For this review, use the dimensioned drawing (mm, ordinates from the lowest corner) and the shaded views. A direction names the side the tool comes from. Give positions to 0.01 mm unless a question says otherwise; leave off trailing zeros. Write each loop counter-clockwise with the first axis right and the second up, starting at its lowest first coordinate (ties: lowest second). Pieces come first, ordered by that corner, then holes.
1) We need section A-A on z = 2. Give the boundary of the cut face in (x, y).
2) We need section D-D on y = 16.5. Give the boundary of the cut face in (x, z), and give its area (3 significant figures).
3) We need section C-C on x = 10.25. Give the boundary of the cut face in (y, z).
4) We need section B-B on x = 5. Give the number of separate pieces and of enclosed holes in the cut face, and give its area (3 significant figures).
5) Machinability: for the marked faces 5, 6, 7, 8 and 9, which of the approach directions +Z, -Z, +X, -X, +Y, -Y give a long, thin tool a straight path to every point of the face, cutting with its end or side? Answer none if there is none.
6) For P1, Ø2, axis at x = 8.5, z = 9, coming from the -Y side; P2, Ø4, axis at x = 8, y = 27.5, coming from the -Z side; P3, Ø0.8, axis at x = 2, z = 13, coming from the -Y side, all flat-tipped, find the tip position at first contact; note any pin that passes through.
7) Wall thickness on line 1 along Z through (x, y) = (5, 31); line 2 along Z through (x, y) = (2.25, 19); line 3 along X through (y, z) = (15, 9.5): over which ranges is each line inside the solid? List them lowest first.
8) Draft analysis for pull direction Y (two halves, no side actions). For the marked faces 1, 2, 3 and 4, state which applies: pulls with the +Y half, pulls with the -Y half, needs draft (parallel to the pull), parting line crosses it, or undercut.
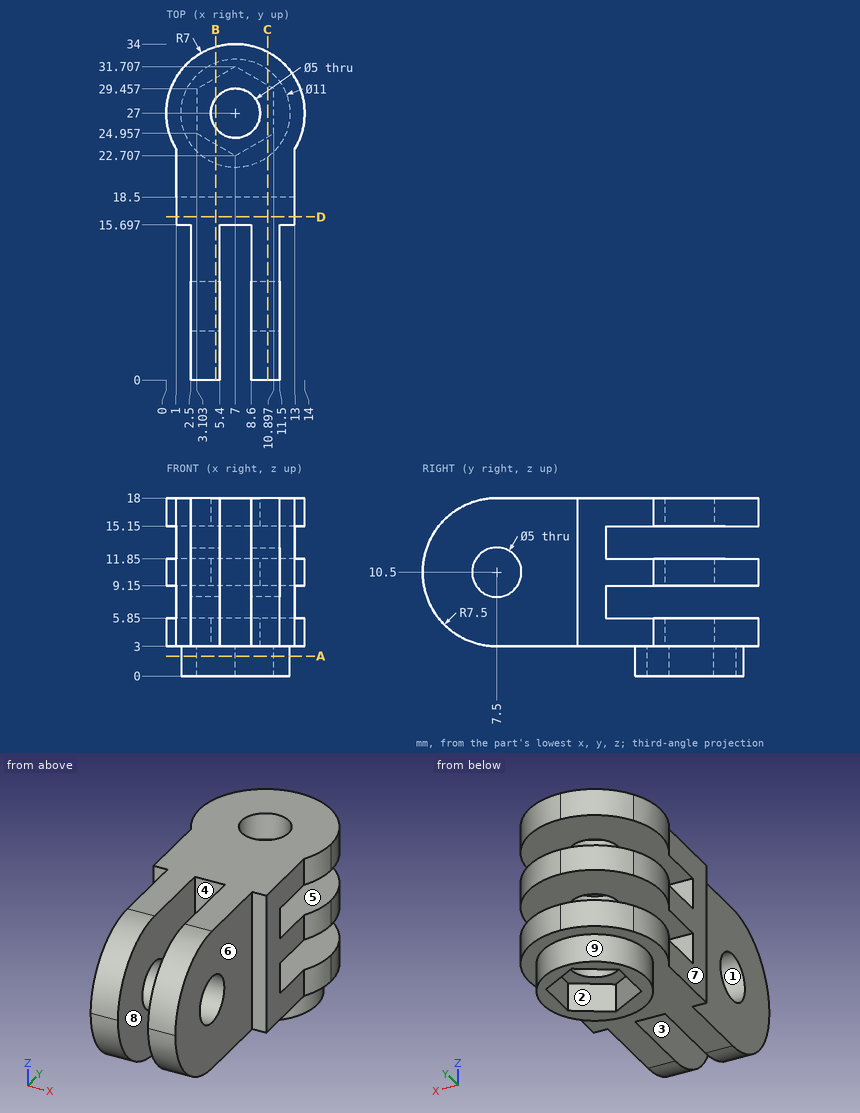
Results list:
1. outline: circle Ø11 at (7, 27); hole (3.1, 24.96) - (7, 22.71) - (10.9, 24.96) - (10.9, 29.46) - (7, 31.71) - (3.1, 29.46) - close
2. outline: (1, 3) - (13, 3) - (13, 18) - (1, 18) - close
2. area: 180 mm2
3. outline: (7.5, 3) - (22.56, 3) - (22.56, 0) - (24.58, 0) - (24.58, 3) - (29.83, 3) - (29.83, 0) - (31.44, 0) - (31.44, 3) - (33.2, 3) - (33.2, 5.85) - (18.5, 5.85) - (18.5, 9.15) - (33.2, 9.15) - (33.2, 11.85) - (18.5, 11.85) - (18.5, 15.15) - (33.2, 15.15) - (33.2, 18) - (7.5, 18) arc R7.5 ccw to start; hole circle Ø5 at (7.5, 10.5)
4. separate pieces: 4
4. enclosed holes: 1
4. area: 347 mm2
5. face 5: +X, -X, +Y
5. face 6: +Z, -Z, +X, -Y
5. face 7: +Z, -Z, -X, -Y
5. face 8: +Z, -Z, -Y
5. face 9: -Z
6. P1: stops at y = 0.02
6. P2: stops at z = 3
6. P3: stops at y = 15.7
7. line 1: z = 0 to 5.85, 9.15 to 11.85, 15.15 to 18
7. line 2: z = 3 to 5.85, 9.15 to 11.85, 15.15 to 18
7. line 3: x = 2.5 to 5.4, 8.6 to 11.5
8. face 1: undercut
8. face 2: undercut
8. face 3: needs draft
8. face 4: pulls with the -Y half
